Here's the drawing with two shaded views (mm, measured from the low corner). I have some questions. Coordinates: 2 decimals unless noted, no trailing zeros. Order: outer loops, then holes, each group sorted by start corner. A loop starts at its lowest first (then second) coordinate and runs counter-clockwise, first axis right, second up. Notation, with made-up numbers: (23.5, 62) -> (82.5, 62) arc R22 ccw to (82.5, 74) -> close; hole circle Ø3 at (21, 84.5). An arc over 180 degrees is marked (long way). Answer in a Markdown table with one row per item. Add a question column.
1. Imagine slicing it at D-D on x = 16.5. Write out the boundary of the cut face in (y, z).
2. We'd pull the mould along Z, two halves only. Please class the marked faces 1, 2 and 3: pulls with the +Z half, pulls with the -Z half, needs draft (parallel to the pull), parting line crosses it, or undercut.
3. Imagine slicing it at C-C on z = 18.5. Write out the boundary of the cut face in (x, y), plus the area to 3 significant figures.
4. If I drill on line 1 along Z through (x, y) = (50, 22.5); line 2 along Z through (x, y) = (51, 12); line 3 along X through (y, z) = (23.5, 8), over which ranges is the centre line in solid material (lowest first)? Write a range as [from, to].
5. Will these pins go through, and if not, where does the flat tip stop? pin 1 (10 mm diameter, centred on x = 27.5, y = 32, fed in from +Z); pin 2 (12 mm diameter, centred on x = 42, y = 24.5, fed in from +Z); pin 3 (2 mm diameter, centred on x = 33.5, y = 30, fed in from -Z).
6. Imagine slicing it at A-A on x = 50. Write out the boundary of the cut face in (y, z), plus the area to 3 significant figures.
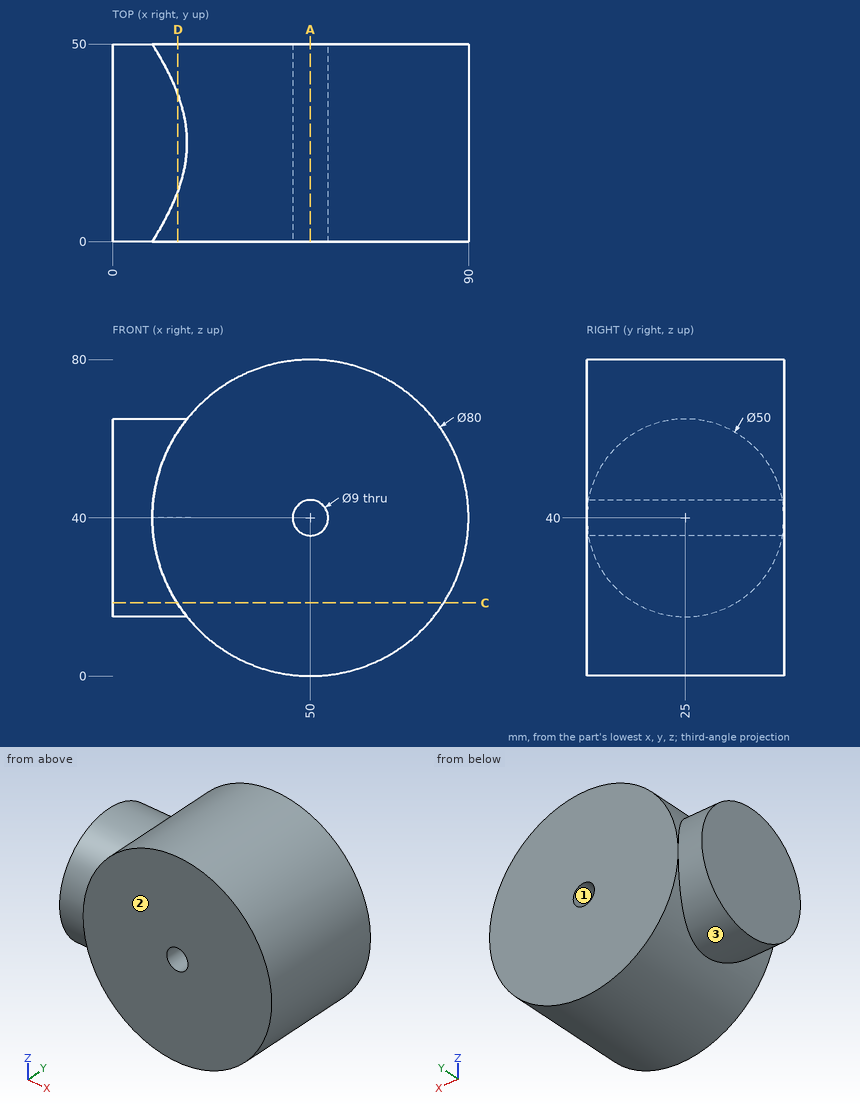
Answers follow:
| question | item | result |
|---|---|---|
| 1 | outline | (0, 18.14) -> (12.87, 18.14) arc R25 ccw to (37.13, 18.14) -> (50, 18.14) -> (50, 61.86) -> (37.13, 61.86) arc R25 ccw to (12.87, 61.86) -> (0, 61.86) -> close |
| 2 | face 1 | undercut |
| 2 | face 2 | needs draft |
| 2 | face 3 | parting line crosses it |
| 3 | outline | (0, 12.24) -> (16.27, 12.24) -> (16.27, 0) -> (83.73, 0) -> (83.73, 50) -> (16.27, 50) -> (16.27, 37.76) -> (0, 37.76) -> close |
| 3 | area | 3,790 mm² |
| 4 | line 1 | z = [0, 35.5], [44.5, 80] |
| 4 | line 2 | z = [0.01, 35.61], [44.39, 79.99] |
| 4 | line 3 | x = [26, 74] |
| 5 | pin 1 | stops at z = 75.97 |
| 5 | pin 2 | stops at z = 79.95 |
| 5 | pin 3 | stops at z = 3.13 |
| 6 | outline | (0, 0) -> (50, 0) -> (50, 35.5) -> (0, 35.5) -> close; (0, 44.5) -> (50, 44.5) -> (50, 80) -> (0, 80) -> close |
| 6 | area | 3,550 mm² |
